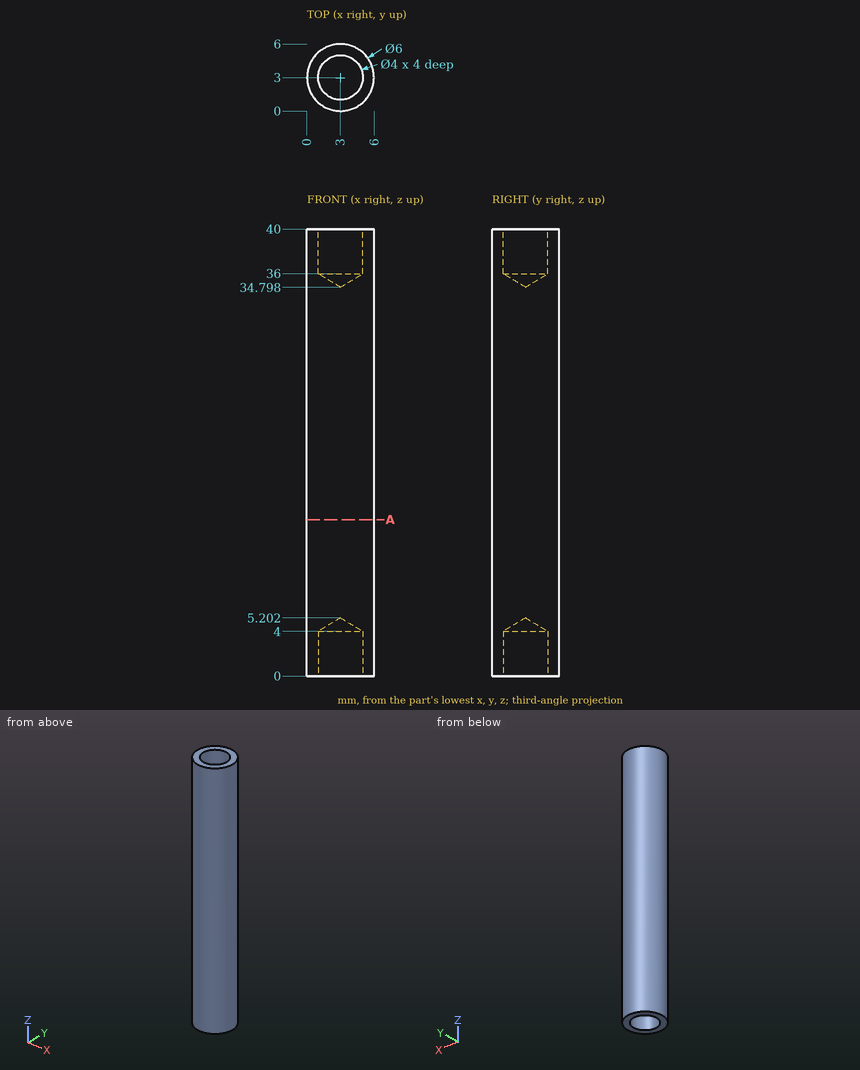
Print and shaded views of the part. All mm, measured from the part's lowest x, y and z. Coordinates: 2 decimals unless noted, no trailing zeros. Order: outer loops, then holes, each group sorted by start corner. A loop starts at its lowest first (then second) coordinate and runs counter-clockwise, first axis right, second up. Notation, with made-up numbers: (34, -26) - (72, -26) arc R30 ccw to (72, 1) - close; hole circle Ø5 at (72, 65.25). An arc over 180 degrees is marked (long way). Return JSON: item names as keys, results as strings. Group by question number.
Item 1: Pin check, flat tip, straight feed: pin 1 (2.5 mm diameter, centred on x = 3, y = 3, fed in from -Z). Stop position of the tip, or through.
Item 2: Cut at A-A (z = 14). List the corners of the cut face in (x, y).
Item 3: Drill centre lines: probe 1 along Y at (x, z) = (3, 1.55); probe 2 along Y at (x, z) = (2.1, 35); probe 3 along Y at (x, z) = (1.7, 27). Where is each one in solid material? Low to high. Write a range as from..to.
Check values:
{
 "1": {"pin 1": "stops at z = 4.45"},
 "2": {"outline": "circle Ø6 at (3, 3)"},
 "3": {"probe 1": "y = 0..1, 5..6", "probe 2": "y = 0.14..5.86", "probe 3": "y = 0.3..5.7"}
}
